Build history of the part. All positions in model axes, mm. Round coordinates to 2 decimals unless told otherwise and drop trailing zeros. Loops run counter-clockwise (first coordinate to the right, second up) from the corner with the lowest first, then second, coordinate; pieces in that order, holes last.
from build123d import *

# Parameters (mm, degrees)
SKETCH4_R           = 3.175
BOSS_EXTRUDE1_DEPTH = 3.175
SKETCH7_R           = 2.0193
CUT_EXTRUDE4_DEPTH  = 5.08


with BuildPart() as part:
    # Sketch4 → Boss-Extrude1 (new body)
    with BuildSketch(Plane.XY):
        Polygon((-38.1, 12.7), (88.9, 12.7), (88.9, -12.7), (88.9, -63.5), (12.7, -63.5), (-12.7, -63.5), (-38.1, -12.7), align=None)
        with Locations((-25.4, 0)):
            Circle(SKETCH4_R, mode=Mode.SUBTRACT)
        Circle(SKETCH4_R, mode=Mode.SUBTRACT)
        with Locations((0, -25.4)):
            Circle(SKETCH4_R, mode=Mode.SUBTRACT)
        with Locations((0, -50.8)):
            Circle(SKETCH4_R, mode=Mode.SUBTRACT)
        with Locations((76.2, 0)):
            Circle(SKETCH4_R, mode=Mode.SUBTRACT)
    extrude(amount=BOSS_EXTRUDE1_DEPTH)

    # Sketch7 → Cut-Extrude4 (cut)
    with BuildSketch(Plane.XY.offset(3.175)):
        with Locations((30.988, -50.8)):
            Circle(SKETCH7_R)
        with Locations((43.688, -50.8)):
            Circle(SKETCH7_R)
        with Locations((56.388, -50.8)):
            Circle(SKETCH7_R)
        with Locations((56.388, 0)):
            Circle(SKETCH7_R)
        with Locations((30.988, 0)):
            Circle(SKETCH7_R)
        with Locations((43.688, 0)):
            Circle(SKETCH7_R)
    extrude(amount=-CUT_EXTRUDE4_DEPTH, mode=Mode.SUBTRACT)


solid = part.part
(1) Pin check, flat tip, straight feed: P1, Ø5, axis at x = 0, y = 0, coming from the +Z side. Stop position of the tip, or through.
Responses:
P1: passes through
(2) Pull direction X, two halves, no side cores. Call faces 1 (the face through (-25.2, -38.5, 1.6)), 2 (the face through (26, -25, 3.175)), 3 (the face through (44.6, -52.6, 1.6)): +X half, -X half, draft (parallel to the pull), parting line (faces both ways), or undercut.
Responses:
face 1: -X half
face 2: draft
face 3: undercut
(3) Probe line 1 (Y direction, x = 0, z = 1.85) (3 decimals); line 2 (Y direction, x = 1.5, z = 1.7); line 3 (Y direction, x = -25.4, z = 1.95) (3 decimals). List the from-to ranges inside material, lowest first.
Responses:
line 1: y = -63.5 to -53.975, -47.625 to -28.575, -22.225 to -3.175, 3.175 to 12.7
line 2: y = -63.5 to -53.6, -48 to -28.2, -22.6 to -2.8, 2.8 to 12.7
line 3: y = -38.1 to -3.175, 3.175 to 12.7
(4) Slice it at B-B on x = 0. List the corners of the cut face in (y, z) (3 decimals).
Responses:
outline: (-63.5, 0) - (-53.975, 0) - (-53.975, 3.175) - (-63.5, 3.175) - close; (-47.625, 0) - (-28.575, 0) - (-28.575, 3.175) - (-47.625, 3.175) - close; (-22.225, 0) - (-3.175, 0) - (-3.175, 3.175) - (-22.225, 3.175) - close; (3.175, 0) - (12.7, 0) - (12.7, 3.175) - (3.175, 3.175) - close
(5) Slice it at C-C on z = 1.2. Count the separate pieces of the cut face and the enclosed holes in it, plus the area to 3 significant figures.
Responses:
separate pieces: 1
enclosed holes: 11
area: 8,800 mm2
(6) Slice it at A-A on y = -25.4. List the corners of the cut face in (x, z) (3 decimals), plus the area to 3 significant figures.
Responses:
outline: (-31.75, 0) - (-3.175, 0) - (-3.175, 3.175) - (-31.75, 3.175) - close; (3.175, 0) - (88.9, 0) - (88.9, 3.175) - (3.175, 3.175) - close
area: 363 mm2
(7) Slice it at D-D on x = -25.4. List the corners of the cut face in (y, z) (3 decimals).
Responses:
outline: (-38.1, 0) - (-3.175, 0) - (-3.175, 3.175) - (-38.1, 3.175) - close; (3.175, 0) - (12.7, 0) - (12.7, 3.175) - (3.175, 3.175) - close
